from build123d import *

# Parameters (mm, degrees)
CUT_EXTRUDE_3_DEPTH      = 10
CUT_EXTRUDE_3_DEPTH_BACK = 10
SKETCH_2_R               = 1.65


with BuildPart() as part:
    # 草图1 → 旋转1 (revolve)
    with BuildSketch(Plane.XY):
        Polygon((0, 0), (-7.7, 0), (-7.7, 1), (-1.5, 4), (-1.5, 8), (0, 8), align=None)
    revolve(axis=Axis((5.3, 12.989187483, 0), (0, -1, 0)))

    # 草图2 → 切除-拉伸3 (cut, two sides: drawn at the far end of the back side and taken through both)
    with BuildSketch(Plane.XY.offset(-CUT_EXTRUDE_3_DEPTH_BACK)):
        with Locations((5.3, 6.4)):
            Circle(SKETCH_2_R)
    extrude(amount=CUT_EXTRUDE_3_DEPTH + CUT_EXTRUDE_3_DEPTH_BACK, mode=Mode.SUBTRACT)


solid = part.part
Source: CAD feature listing. Evaluate the final solid. Frame: model axes, mm. A direction names the side the tool comes from. Give positions to 0.01 mm unless a question says otherwise; leave off trailing zeros. Loops run counter-clockwise (first coordinate to the right, second up) from the corner with the lowest first, then second, coordinate; pieces in that order, holes last. Notation, with made-up numbers: (70.5, -17.75) -> (121.5, -17.75) arc R26 ccw to (121.5, 20.25) -> close; hole circle Ø10 at (48.5, 14.5). An arc over 180 degrees is marked (long way). Use a Markdown table: item, result. Add a question column.
1) Section query A-A, the plane x = 5.3. Return the cut outline in (y, z), then the cut area to 4 significant figures.
2) Line query: line 1 along X through (y, z) = (5.5, 0); line 2 along X through (y, z) = (0.5, -0.25); line 3 along Y through (x, z) = (5.3, 5.8). Output: solid intervals per line, ascending. Write a range as [from, to].
3) Section query C-C, the plane y = 7.25. Return the cut outline in (x, z), then the cut area to 3 significant figures.
4) Section query B-B, the plane z = 0. Return the cut outline in (x, y).
5) Reachability of faces 1 (the face through (15.616, 0.507, 7.91)), 2 (the face through (2.16, 6.03, 6.03)) from +Z, -Z, +X, -X, +Y, -Y: full face, straight path, thin tool, end or side. Return the list, or none.
6) Pull-direction query (X, two-part tool) for faces 3 (the face through (-0.2, 8, 0)), 4 (the face through (5.23, 4.75, -5.93)), 5 (the face through (10.935, 3.854, 4.321)); classes: +X half, -X half, draft (parallel to the pull), parting line (faces both ways), or undercut.
7) Section query D-D, the plane y = 1.75. Return the cut outline in (x, z).
8) First-contact query: pin 1 (4 mm diameter, centred on x = -2.5, y = 2.5, fed in from +Z); pin 2 (4.5 mm diameter, centred on x = 5.3, y = 6.4, fed in from -Z); pin 3 (2 mm diameter, centred on x = 13, y = 1.5, fed in from +Z). Flat tips, straight axial feed; report the tip coordinate or a pass-through.
Numbers:
| question | item | result |
|---|---|---|
| 1 | outline | (0, -13) -> (1, -13) -> (4, -6.8) -> (4.75, -6.8) -> (4.75, -5.3) -> (0, -5.3) -> close; (0, 5.3) -> (4.75, 5.3) -> (4.75, 6.8) -> (4, 6.8) -> (1, 13) -> (0, 13) -> close |
| 1 | area | 45.25 mm2 |
| 2 | line 1 | x = [-1.5, 0], [10.6, 12.1] |
| 2 | line 2 | x = [-7.7, 0.01], [10.59, 18.3] |
| 2 | line 3 | y = [0, 4.75] |
| 3 | outline | (3.89, -6.65) -> (3.89, -5.11) arc R5.3 cw to (3.89, 5.11) -> (3.89, 6.65) arc R6.8 ccw to start; (6.71, -6.65) arc R6.8 ccw to (6.71, 6.65) -> (6.71, 5.11) arc R5.3 cw to (6.71, -5.11) -> close |
| 3 | area | 48.5 mm2 |
| 4 | outline | (-7.7, 0) -> (0, 0) -> (0, 8) -> (-1.5, 8) -> (-1.5, 4) -> (-7.7, 1) -> close; (10.6, 0) -> (18.3, 0) -> (18.3, 1) -> (12.1, 4) -> (12.1, 8) -> (10.6, 8) -> close |
| 5 | face 1 | +Y, -Y |
| 5 | face 2 | +Y |
| 6 | face 3 | draft |
| 6 | face 4 | undercut |
| 6 | face 5 | parting line |
| 7 | outline | circle Ø22.9 at (5.3, 0); hole circle Ø10.6 at (5.3, 0) |
| 8 | pin 1 | stops at z = 11.27 |
| 8 | pin 2 | stops at z = -6.8 |
| 8 | pin 3 | stops at z = 11.06 |
